Model file for the job. Use its own axes, mm. Give positions to 0.01 mm unless a question says otherwise; leave off trailing zeros. Return JSON: item names as keys, results as strings. Group by question number.
1. Slice it at A-A on y = 0.6. Give the number of separate pieces and of enclosed holes in the cut face, then the cut area to 3 significant figures.
2. Two-plate mould, pull along Z, no slides. Class faces 1 (the face through (-1, 0, -15)), 2 (the face through (75.65, 1.48, -52.47)), 3 (the face through (-89.439, 1.521, 154.336)): released by +Z, released by -Z, zero draft, split by the parting line, or undercut.
3. Wall check: probe 1 along Z at (x, y) = (-77, 2.15); probe 2 along Z at (x, y) = (77, 2.75); probe 3 along X at (y, z) = (2.9, -52). Give the ranges that are in metal, low to high. Write a range as [from, to].
4. Pin check, flat tips, straight feed: pin 1 (4 mm diameter, centred on x = 86.65, z = -12.48, fed in from -Y); pin 2 (1.5 mm diameter, centred on x = -86, y = 1.5, fed in from -Z); pin 3 (0.9 mm diameter, centred on x = 85, y = 1.5, fed in from -Z). Stop position of each tip, or through.
from build123d import *

# Parameters (mm, degrees)
SKETCH1_W                 = 158.69
SKETCH1_H                 = 25
BOSS_EXTRUDE1_DEPTH       = 3
FILLET1_R                 = 10
FILLET2_R                 = 6
F_4_CLEARANCE_HOLE1_D     = 3.2639
F_4_CLEARANCE_HOLE1_DEPTH = 3
F_4_CLEARANCE_HOLE1_TIP   = 0.980574487
FILLET3_R                 = 2


with BuildPart() as part:
    # Sketch1 → Boss-Extrude1 (new body)
    with BuildSketch(Plane(origin=(0, 0, 0), x_dir=(1, 0, 0), z_dir=(0, 1, 0))):
        with BuildLine():
            Line((-91.15, 34.109827366), (-82.15, 34.109827366))
            ThreePointArc((-82.15, 34.109827366), (-75.65, 27.609827366), (-82.15, 21.109827366))
            Line((-82.15, 21.109827366), (-91.15, 21.109827366))
            Line((-91.15, 21.109827366), (-91.15, -46.140172634))
            Line((-91.15, -46.140172634), (-82.15, -46.140172634))
            ThreePointArc((-82.15, -46.140172634), (-75.65, -52.640172634), (-82.15, -59.140172634))
            Line((-82.15, -59.140172634), (-91.15, -59.140172634))
            Line((-91.15, -59.140172634), (-91.15, -126.390172634))
            Line((-91.15, -126.390172634), (-82.15, -126.390172634))
            ThreePointArc((-82.15, -126.390172634), (-75.65, -132.890172634), (-82.15, -139.390172634))
            Line((-82.15, -139.390172634), (-91.15, -139.390172634))
            Line((-91.15, -139.390172634), (-91.15, -156.140172634))
            Line((-91.15, -156.140172634), (91.15, -156.140172634))
            Line((91.15, -156.140172634), (91.15, -114.390172634))
            Line((91.15, -114.390172634), (82.15, -114.390172634))
            ThreePointArc((82.15, -114.390172634), (75.65, -107.890172634), (82.15, -101.390172634))
            Line((82.15, -101.390172634), (91.15, -101.390172634))
            Line((91.15, -101.390172634), (91.15, -34.140172634))
            Line((91.15, -34.140172634), (82.15, -34.140172634))
            ThreePointArc((82.15, -34.140172634), (75.65, -27.640172634), (82.15, -21.140172634))
            Line((82.15, -21.140172634), (91.15, -21.140172634))
            Line((91.15, -21.140172634), (91.15, 46.109827366))
            Line((91.15, 46.109827366), (82.15, 46.109827366))
            ThreePointArc((82.15, 46.109827366), (75.65, 52.609827366), (82.15, 59.109827366))
            Line((82.15, 59.109827366), (91.15, 59.109827366))
            Line((91.15, 59.109827366), (91.15, 126.359827366))
            Line((91.15, 126.359827366), (82.15, 126.359827366))
            ThreePointArc((82.15, 126.359827366), (75.65, 132.859827366), (82.15, 139.359827366))
            Line((82.15, 139.359827366), (91.15, 139.359827366))
            Line((91.15, 139.359827366), (91.15, 156.140172634))
            Line((91.15, 156.140172634), (67.54, 156.140172634))
            Line((67.54, 156.140172634), (-91.15, 156.140172634))
            Line((-91.15, 156.140172634), (-91.15, 114.359827366))
            Line((-91.15, 114.359827366), (-82.15, 114.359827366))
            ThreePointArc((-82.15, 114.359827366), (-75.65, 107.859827366), (-82.15, 101.359827366))
            Line((-82.15, 101.359827366), (-91.15, 101.359827366))
            Line((-91.15, 101.359827366), (-91.15, 34.109827366))
        make_face()
        with Locations((-11.805, 168.640172634)):
            Rectangle(SKETCH1_W, SKETCH1_H)
    extrude(amount=BOSS_EXTRUDE1_DEPTH)

    # Fillet1
    fillet1_edges = [part.edges().sort_by_distance(p)[0] for p in [
        (-91.15, 1.5, -181.140172634),
    ]]
    fillet(fillet1_edges, radius=FILLET1_R)

    # Fillet2
    fillet2_edges = [part.edges().sort_by_distance(p)[0] for p in [
        (91.15, 1.5, 156.140172634),
        (-91.15, 1.5, 156.140172634),
        (91.15, 1.5, -156.140172634),
    ]]
    fillet(fillet2_edges, radius=FILLET2_R)

    # #4 Clearance Hole1
    with Locations(Plane(origin=(0, 3, 0), x_dir=(1, 0, 0), z_dir=(0, 1, 0))):
        with Locations((86.65, 148.140172634), (-86.65, -148.140172634), (-86.65, -12.515172634), (-86.65, 148.140172634), (86.65, 12.484827366), (86.65, -148.140172634)):
            Hole(F_4_CLEARANCE_HOLE1_D / 2, depth=F_4_CLEARANCE_HOLE1_DEPTH)
            with Locations((0, 0, -(F_4_CLEARANCE_HOLE1_DEPTH + F_4_CLEARANCE_HOLE1_TIP / 2))):  # 118° drill point
                Cone(0, F_4_CLEARANCE_HOLE1_D / 2, F_4_CLEARANCE_HOLE1_TIP, mode=Mode.SUBTRACT)

    # Fillet3
    fillet3_edges = [part.edges().sort_by_distance(p)[0] for p in [
        (67.54, 1.5, -181.140172634),
        (91.15, 1.5, -126.359827366),
        (91.15, 1.5, -59.109827366),
        (91.15, 1.5, -46.109827366),
        (91.15, 1.5, 21.140172634),
        (91.15, 1.5, 34.140172634),
        (91.15, 1.5, 101.390172634),
        (91.15, 1.5, 114.390172634),
        (-91.15, 1.5, 139.390172634),
        (-91.15, 1.5, 126.390172634),
        (-91.15, 1.5, 59.140172634),
        (-91.15, 1.5, 46.140172634),
        (-91.15, 1.5, -21.109827366),
        (-91.15, 1.5, -34.109827366),
        (-91.15, 1.5, -101.359827366),
        (-91.15, 1.5, -114.359827366),
        (91.15, 1.5, -139.359827366),
    ]]
    fillet(fillet3_edges, radius=FILLET3_R)


solid = part.part
Result:
{
 "1": {"separate pieces": "1", "enclosed holes": "6", "area": "59,300 mm2"},
 "2": {"face 1": "zero draft", "face 2": "undercut", "face 3": "released by +Z"},
 "3": {"probe 1": "z = [-181.14, -111.83], [-103.89, -31.58], [-23.64, 48.67], [56.61, 128.92], [136.86, 156.14]", "probe 2": "z = [-156.14, -136.83], [-128.89, -56.58], [-48.64, 23.67], [31.61, 103.92], [111.86, 156.14]", "probe 3": "x = [-91.15, 75.68]"},
 "4": {"pin 1": "stops at y = 0", "pin 2": "stops at z = -180.26", "pin 3": "stops at z = -156.14"}
}
